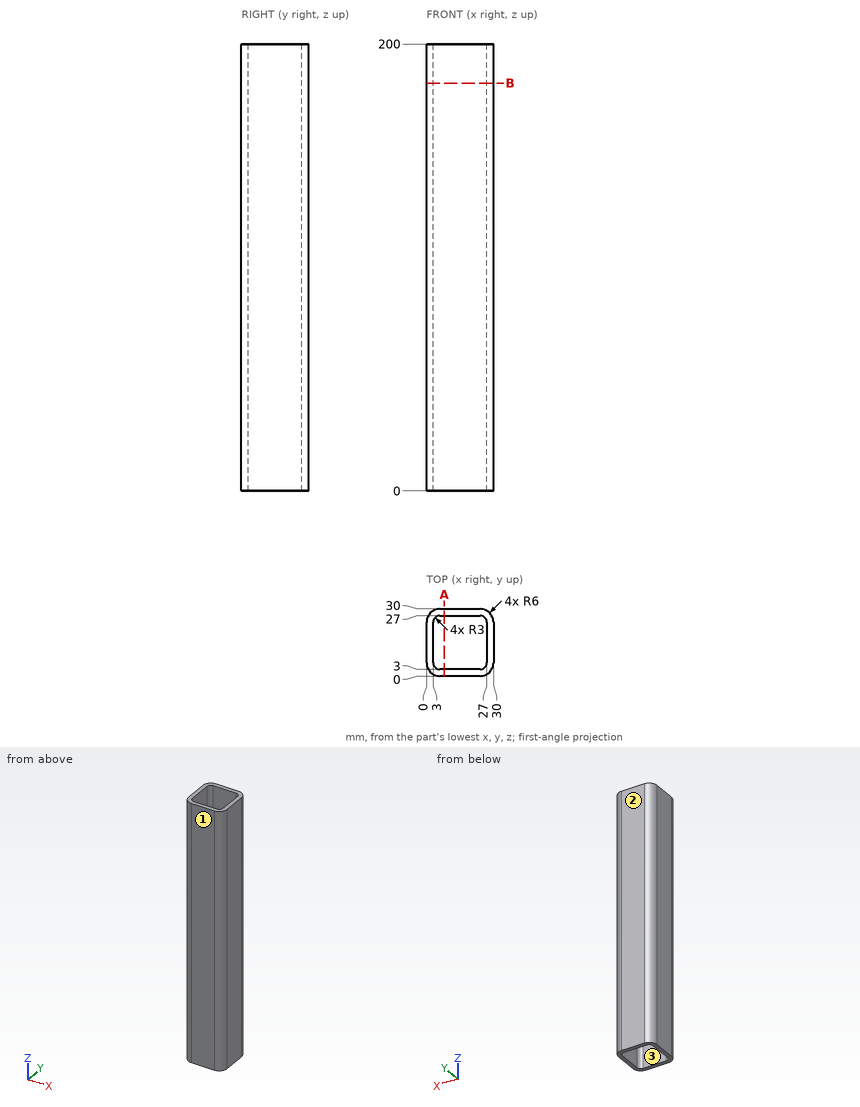
Geometry: see drawing. Coordinates: mm, zero at the bounding-box minimum. Coordinates: 2 decimals unless noted, no trailing zeros. Loops run counter-clockwise (first coordinate to the right, second up) from the corner with the lowest first, then second, coordinate; pieces in that order, holes last. Notation, with made-up numbers: (-6, 80) -> (6, 80) arc R15 ccw to (6, 89) -> close; hole circle Ø10 at (13.5, 55). An arc over 180 degrees is marked (long way). Write item = value, one per line. Start each with the question number.
Item 1: Cut plane A-A, the plane x = 8. Return loops of the section in (y, z), plus the area to 3 significant figures.
Item 2: Cut plane B-B, the plane z = 182.5. Return loops of the section in (x, y).
Item 3: Mould query, pull axis Y, two halves, no side actions, for the marked faces 1, 2 and 3. Classes: pulls with the +Y half, pulls with the -Y half, needs draft (parallel to the pull), parting line crosses it, or undercut.
Item 4: Material intervals for line 1 (X direction, y = 12, z = 64); line 2 (X direction, y = 26.5, z = 110.5), sorted ascending.
Ans:
q1.outline = (0, 0) -> (3, 0) -> (3, 200) -> (0, 200) -> close; (27, 0) -> (30, 0) -> (30, 200) -> (27, 200) -> close
q1.area = 1,200 mm²
q2.outline = (0, 6) arc R6 ccw to (6, 0) -> (24, 0) arc R6 ccw to (30, 6) -> (30, 24) arc R6 ccw to (24, 30) -> (6, 30) arc R6 ccw to (0, 24) -> close; hole (3, 6) arc R3 ccw to (6, 3) -> (24, 3) arc R3 ccw to (27, 6) -> (27, 24) arc R3 ccw to (24, 27) -> (6, 27) arc R3 ccw to (3, 24) -> close
q3.face_1 = pulls with the -Y half
q3.face_2 = pulls with the +Y half
q3.face_3 = undercut
q4.line_1 = 0 to 3, 27 to 30
q4.line_2 = 0.55 to 4.34, 25.66 to 29.45
